Autodesk Inventor part; units mm, degrees
ref_plane "YZ Plane" through (0, 0, 0) normal (1, 0, 0) x (0, 1, 0)
ref_plane "XZ Plane" through (0, 0, 0) normal (0, 1, 0) x (-1, 0, 0)
ref_plane "XY Plane" through (0, 0, 0) normal (0, 0, 1) x (1, 0, 0)
sketch "Sketch1" plane through (0, 0, 0) normal (0, 0, 1) x (1, 0, 0)
  circle A0 centre (0, 0) radius 2.15
  circle A1 centre (0, 0) radius 2.75
  line L0 (0, 3.1754) -> (2.75, 1.5877)
  line L1 (2.75, 1.5877) -> (2.75, -1.5877)
  line L2 (2.75, -1.5877) -> (0, -3.1754)
  line L3 (0, -3.1754) -> (-2.75, -1.5877)
  line L4 (-2.75, -1.5877) -> (-2.75, 1.5877)
  line L5 (-2.75, 1.5877) -> (0, 3.1754)
  dimension "d0" = 4.3
  dimension "d1" = 5.5
extrude "Extrusion1" add sketch "Sketch1" along normal mid plane 5
sketch "Sketch2" plane through (0, 0, 0) normal (1, 0, 0) x (0, 1, 0)
  line L0 (3.1754, 2.5) -> (1.5877, 2.5)
  line L1 (3.1754, 2.5) -> (3.1754, 1.75)
  line L2 (3.1754, 2.5) -> (2.4254, 2.5)
  line L3 (2.4254, 2.5) -> (3.1754, 1.75)
  line L4 (1.5877, 2.5) -> (-1.5877, 2.5)
  line L5 (0, 2.5) -> (0, -2.5) construction
  line L6 (2.15, -2.5) -> (-2.15, -2.5)
  line L7 (1.5877, -2.5) -> (3.1754, -2.5)
  line L8 (3.1754, -2.5) -> (3.1754, -1.75)
  line L9 (3.1754, -2.5) -> (2.4254, -2.5)
  line L10 (2.4254, -2.5) -> (3.1754, -1.75)
  point P0 (0, 0)
  dimension "d4" = 0.75
  dimension "d5" = 0.75
  dimension "d6" = 0.75
  dimension "d7" = 0.75
revolve "Revolution1" cut sketch "Sketch2" angle 360 about axis through (0, 0, 2.5) along (0, 0, -1)
thread "Thread3"
properties part number "L3 Part 7" material "Stainless Steel"
The listing builds one solid part. Answer for the finished solid, in the listing's coordinates (mm). Coordinates: 2 decimals unless noted, no trailing zeros. Order: outer loops, then holes, each group sorted by start corner. A loop starts at its lowest first (then second) coordinate and runs counter-clockwise, first axis right, second up. Notation, with made-up numbers: (-10.5, 22.5) -> (30.5, 22.5) arc R16 cw to (30.5, 51.5) -> close; hole circle Ø8 at (89, -15.75). An arc over 180 degrees is marked (long way). Answer in a Markdown table with one row per item. Add a question column.
Item 1: Each of these flat-tipped pins is pushed along its axis until it touches: P1, Ø2, axis at y = -2, z = -2, coming from the +X side; P2, Ø1, axis at x = -1.5, z = -0.5, coming from the +Y side. Where does it stop, or does it pass through?
Item 2: Determine the mould class of faces 1 (the face through (1.36, 2.39, -0.03)), 2 (the face through (-1.36, -2.39, -0.03)), 3 (the face through (-2.15, -0.09, -0.04)) for opening direction Y: +Y half, -Y half, draft (parallel to the pull), parting line (faces both ways), or undercut.
Item 3: Find the intervals of material crossed by L1, parallel to X at y = -1, z = -0.3; L2, parallel to Y at x = -1.35, z = 1.55; L3, parallel to Y at x = 0.6, z = 1.3, in increasing order. Write a range as from..to.
Item 4: Find section B-B (z = -0.3). Write down the section's boundary in (x, y).
Item 5: Find section A-A (y = 0). Write down the section's boundary in (x, z), then the cut area to 3 significant figures.
Result set:
| question | item | result |
|---|---|---|
| 1 | P1 | stops at x = 2.75 |
| 1 | P2 | stops at y = 2.6 |
| 2 | face 1 | +Y half |
| 2 | face 2 | -Y half |
| 2 | face 3 | undercut |
| 3 | L1 | x = -2.75..-1.9, 1.9..2.75 |
| 3 | L2 | y = -2.4..-1.67, 1.67..2.4 |
| 3 | L3 | y = -2.83..-2.06, 2.06..2.83 |
| 4 | outline | (-2.75, -1.59) -> (0, -3.18) -> (2.75, -1.59) -> (2.75, 1.59) -> (0, 3.18) -> (-2.75, 1.59) -> close; hole circle Ø4.3 at (0, 0) |
| 5 | outline | (-2.75, -2.18) -> (-2.43, -2.5) -> (-2.15, -2.5) -> (-2.15, 2.5) -> (-2.43, 2.5) -> (-2.75, 2.18) -> close; (2.15, -2.5) -> (2.43, -2.5) -> (2.75, -2.18) -> (2.75, 2.18) -> (2.43, 2.5) -> (2.15, 2.5) -> close |
| 5 | area | 5.79 mm² |
